Here's the drawing with two shaded views (mm, measured from the low corner). I have some questions. Round coordinates to 2 decimals unless told otherwise and drop trailing zeros. Write each loop counter-clockwise with the first axis right and the second up, starting at its lowest first coordinate (ties: lowest second). Pieces come first, ordered by that corner, then holes. Notation, with made-up numbers: (7.25, 2) - (25.25, 2) arc R23 cw to (25.25, 24) - close; hole circle Ø7 at (-6.5, 73.5). An arc over 180 degrees is marked (long way). Return JSON: item names as keys, results as strings. Group by question number.
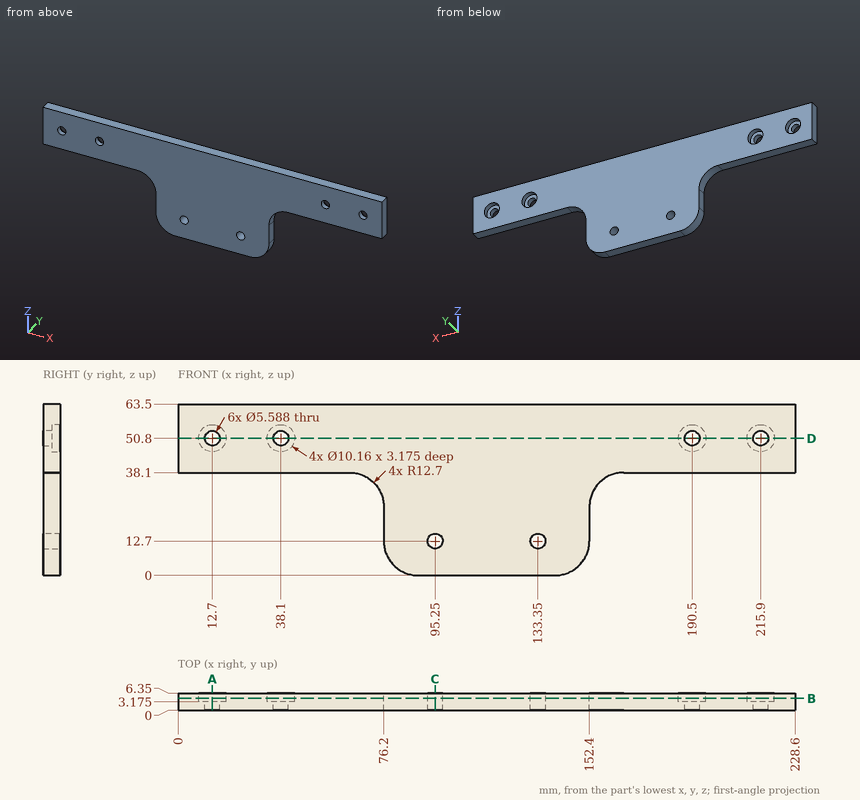
1) Imagine slicing it at B-B (y = 4.5). Please give me the cut outline in (x, z).
2) Will these pins go through, and if not, where does the flat tip stop? pin 1 Ø13 at (x, z) = (38.1, 50.8) entering from +Y; pin 2 Ø1.5 at (y, z) = (4.5, 24) entering from -X; pin 3 Ø1.9 at (x, y) = (200, 3) entering from -Z; pin 4 Ø5 at (x, z) = (14.5, 52) entering from +Y (3 decimals).
3) Imagine slicing it at D-D (z = 50.8). Give the number of separate pieces and of enclosed holes in the cut face, plus the area to 3 significant figures.
4) I need wall thicknesses on line 1 along X through (y, z) = (0.85, 50.8); line 2 along X through (y, z) = (3.25, 12.7); line 3 along Z through (x, y) = (190.5, 4.75). Which ranges of each line are inside material? Lowest first, please.
5) Imagine slicing it at A-A (x = 12.7). Please give me the cut outline in (y, z) (3 decimals).
6) Imagine slicing it at C-C (x = 95.25). Please give me the cut outline in (y, z).
Results found:
{
 "1": {"outline": "(0, 38.1) - (63.5, 38.1) arc R12.7 cw to (76.2, 25.4) - (76.2, 12.7) arc R12.7 ccw to (88.9, 0) - (139.7, 0) arc R12.7 ccw to (152.4, 12.7) - (152.4, 25.4) arc R12.7 cw to (165.1, 38.1) - (228.6, 38.1) - (228.6, 63.5) - (0, 63.5) - close; hole circle Ø10.16 at (12.7, 50.8); hole circle Ø10.16 at (38.1, 50.8); hole circle Ø5.59 at (95.25, 12.7); hole circle Ø5.59 at (133.35, 12.7); hole circle Ø10.16 at (190.5, 50.8); hole circle Ø10.16 at (215.9, 50.8)"},
 "2": {"pin 1": "stops at y = 6.35", "pin 2": "stops at x = 76.2", "pin 3": "stops at z = 38.1", "pin 4": "stops at y = 3.175"},
 "3": {"separate pieces": "5", "enclosed holes": "0", "area": "1,250 mm²"},
 "4": {"line 1": "x = 0 to 9.91, 15.49 to 35.31, 40.89 to 187.71, 193.29 to 213.11, 218.69 to 228.6", "line 2": "x = 76.2 to 92.46, 98.04 to 130.56, 136.14 to 152.4", "line 3": "z = 38.1 to 45.72, 55.88 to 63.5"},
 "5": {"outline": "(0, 38.1) - (6.35, 38.1) - (6.35, 45.72) - (3.175, 45.72) - (3.175, 48.006) - (0, 48.006) - close; (0, 53.594) - (3.175, 53.594) - (3.175, 55.88) - (6.35, 55.88) - (6.35, 63.5) - (0, 63.5) - close"},
 "6": {"outline": "(0, 0) - (6.35, 0) - (6.35, 9.91) - (0, 9.91) - close; (0, 15.49) - (6.35, 15.49) - (6.35, 63.5) - (0, 63.5) - close"}
}
